from build123d import *

# Parameters (mm, degrees)
SKETCH_1_W               = 39.5
SKETCH_1_H               = 14.5
EXTRUDE_1_DEPTH          = 40
SKETCH_6_W               = 80
SKETCH_6_H               = 160
EXTRUDE_2_DEPTH          = 10
EXTRUDE_3_DEPTH          = 10
SKETCH_8_W               = 40
SKETCH_8_H               = 60
CUT_EXTRUDE_1_DEPTH      = 10
SKETCH_9_W               = 20
SKETCH_9_H               = 8
CUT_EXTRUDE_3_DEPTH      = 10
CUT_EXTRUDE_4_DEPTH      = 158.764612799
CUT_EXTRUDE_4_DEPTH_BACK = 1
CUT_EXTRUDE_5_DEPTH      = 1


with BuildPart() as part:
    # 草图1 → 凸台-拉伸1 (new body)
    with BuildSketch(Plane.XY):
        Rectangle(SKETCH_1_W, SKETCH_1_H)
    extrude(amount=EXTRUDE_1_DEPTH)

    # 草图6 → 凸台-拉伸2 (add)
    with BuildSketch(Plane(origin=(0, 15.03668382, 28.054947672), x_dir=(1, 0, 0), z_dir=(0, 0.4723983215829414, 0.8813851744643881))):
        with Locations((0, 22.485349826)):
            Rectangle(SKETCH_6_W, SKETCH_6_H)
    extrude(amount=EXTRUDE_2_DEPTH)

    # 草图7 → 凸台-拉伸3 (add)
    with BuildSketch(Plane(origin=(0, 19.760667036, 36.868799416), x_dir=(1, 0, 0), z_dir=(0, 0.4723983215829416, 0.881385174464388))):
        Polygon((-35, -52.514650174), (35, -52.514650174), (35, 102.485349826), (40, 102.485349826), (40, -57.514650174), (-40, -57.514650174), (-40, 102.485349826), (-35, 102.485349826), align=None)
    extrude(amount=EXTRUDE_3_DEPTH)

    # 草图8 → 切除-拉伸1 (cut)
    with BuildSketch(Plane(origin=(0, 19.760667036, 36.868799416), x_dir=(1, 0, 0), z_dir=(0, 0.47239832158294137, 0.8813851744643881))):
        with Locations((-10, 67.485349826)):
            Rectangle(SKETCH_8_W, SKETCH_8_H)
    extrude(amount=-CUT_EXTRUDE_1_DEPTH, mode=Mode.SUBTRACT)

    # 草图9 → 切除-拉伸3 (cut)
    with BuildSketch(Plane(origin=(0, -50.692559978, 27.169824208), x_dir=(1, 0, 0), z_dir=(0, -0.881385174464388, 0.47239832158294154))):
        with Locations((-0.027304515, 45.830519147)):
            Rectangle(SKETCH_9_W, SKETCH_9_H)
    extrude(amount=-CUT_EXTRUDE_3_DEPTH, mode=Mode.SUBTRACT)

    # 草图10 → 切除-拉伸4 (cut, two sides: drawn at the far end of the back side and taken through both)
    with BuildSketch(Plane.ZY.offset(40).offset(-CUT_EXTRUDE_4_DEPTH_BACK)):
        Polygon((235.352563611, -333.840604393), (71.001566503, -27.199946201), (-4.58216495, 113.821681713), (-3.612641258, 114.341319867), (71.971090195, -26.680308047), (236.322087302, -333.320966239), (565.024081517, -946.602282623), (564.054557825, -947.121920777), align=None)
    extrude(amount=CUT_EXTRUDE_4_DEPTH + CUT_EXTRUDE_4_DEPTH_BACK, mode=Mode.SUBTRACT)

    # 草图11 → 切除-拉伸5 (cut)
    with BuildSketch(Plane(origin=(40, 0, 0), x_dir=(0, 0, -1), z_dir=(1, 0, 0))):
        Polygon((3.612641258, 114.341319867), (-71.971090195, -26.680308047), (-71.001566503, -27.199946201), (4.58216495, 113.821681713), align=None)
    extrude(amount=-CUT_EXTRUDE_5_DEPTH, mode=Mode.SUBTRACT)


solid = part.part
Build history of the part. All positions in model axes, mm. A direction names the side the tool comes from. Coordinates: 2 decimals unless noted, no trailing zeros. Order: outer loops, then holes, each group sorted by start corner. A loop starts at its lowest first (then second) coordinate and runs counter-clockwise, first axis right, second up. Notation, with made-up numbers: (-37.5, -32) - (-30.5, -32) arc R15 ccw to (-30.5, -20) - close; hole circle Ø6 at (-9.75, 43). An arc over 180 degrees is marked (long way). Put each result on its own line as item: value.
1. Saw through at B-B (z = 15). Write the cut outline in (x, y).
Answer sheet:
outline: (-40, 39.39) - (40, 39.39) - (40, 77.29) - (39, 77.29) - (39, 79.61) - (40, 79.61) - (40, 81.73) - (35, 81.73) - (35, 60.56) - (10, 60.56) - (10, 50.57) - (-30, 50.57) - (-30, 60.56) - (-35, 60.56) - (-35, 81.73) - (-40, 81.73) - (-40, 79.61) - (-39, 79.61) - (-39, 77.29) - (-40, 77.29) - close; (-19.75, -7.25) - (19.75, -7.25) - (19.75, 7.25) - (-19.75, 7.25) - close
2. Saw through at A-A (x = -14). Write the cut outline in (y, z), and give its area (3 significant figures).
Answer sheet:
outline: (-35.66, 55.22) - (-7.25, 40) - (-7.25, 0) - (7.25, 0) - (7.25, 32.23) - (48.08, 10.35) - (52.8, 19.16) - (-26.52, 61.68) - (-21.8, 70.49) - (-26.21, 72.85) - close; (100.96, -18) - (105.37, -20.36) - (110.09, -11.55) - (105.68, -9.18) - close
area: 1,570 mm^2
3. Saw through at C-C (x = 5). Write the cut outline in (y, z).
Answer sheet:
outline: (-35.66, 55.22) - (-7.25, 40) - (-7.25, 0) - (7.25, 0) - (7.25, 32.23) - (48.08, 10.35) - (52.8, 19.16) - (-30.93, 64.04) - close; (-27.15, 71.09) - (-22.75, 68.73) - (-21.8, 70.49) - (-26.21, 72.85) - close; (100.96, -18) - (105.37, -20.36) - (110.09, -11.55) - (105.68, -9.18) - close
4. Drop flat-ended pins along their axis: P1, Ø20, axis at x = -2, z = 19.5, coming from the -Y side; P2, Ø16, axis at y = 1, z = 22, coming from the +X side; P3, Ø16, axis at y = -1.5, z = 27, coming from the -X side. Give the stop position or say it passes through.
Answer sheet:
P1: stops at y = -7.25
P2: stops at x = 19.75
P3: stops at x = -19.75
5. Tool access for faces 1 (the face through (-10.28, 50.471, 14.816)), 2 (the face through (-0.167, -24.98, 69.925)), 3 (the face through (-39, 49, 31)): list every direction of +Z, -Z, +X, -X, +Y, -Y with a clear straight run to the whole face (end or side of a thin tool).
Answer sheet:
face 1: -Z, +Y
face 2: -Y
face 3: -X
6. Probe line 1 along X through (y, z) = (28, 36.5); line 2 along X through (y, z) = (64.5, 6.5); line 3 along Y through (x, z) = (16.5, 11.5). List the from-to ranges inside material, lowest first. Write a range as [from, to].
Answer sheet:
line 1: x = [-40, -35], [35, 40]
line 2: x = [-40, -30], [10, 40]
line 3: y = [-7.25, 7.25], [45.92, 67.09]
7. Saw through at D-D (y = 65). Write the cut outline in (x, z), and give its area (3 significant figures).
Answer sheet:
outline: (-40, 1.28) - (-30, 1.28) - (-30, 12.62) - (-35, 12.62) - (-35, 23.97) - (-40, 23.97) - (-40, 22.83) - (-39, 22.83) - (-39, 21.58) - (-40, 21.58) - close; (10, 1.28) - (40, 1.28) - (40, 21.58) - (39, 21.58) - (39, 22.83) - (40, 22.83) - (40, 23.97) - (35, 23.97) - (35, 12.62) - (10, 12.62) - close
area: 565 mm^2
8. Pull direction X, two halves, no side cores. Call faces 4 (the face through (-40, 38, 26)), 5 (the face through (10, 77, 1)), 6 (the face through (-0.56, 20.173, 25.302)): pulls with the +X half, pulls with the -X half, needs draft (parallel to the pull), parting line crosses it, or undercut.
Answer sheet:
face 4: pulls with the -X half
face 5: undercut
face 6: needs draft
